```python
from build123d import *

# Parameters (mm, degrees)
ESQUISSE1_W        = 110
ESQUISSE1_H        = 50
ESQUISSE1_W_2      = 10
ESQUISSE1_H_2      = 10
BOSS_EXTRU_1_DEPTH = 4
CONG_1_R           = 3


with BuildPart() as part:
    # Esquisse1 → Boss.-Extru.1 (new body)
    with BuildSketch(Plane.XY):
        Rectangle(ESQUISSE1_W, ESQUISSE1_H)
        with Locations((-20, 0)):
            Rectangle(ESQUISSE1_W_2, ESQUISSE1_H_2, mode=Mode.SUBTRACT)
        with Locations((-40, 0)):
            Rectangle(ESQUISSE1_W_2, ESQUISSE1_H_2, mode=Mode.SUBTRACT)
        Rectangle(ESQUISSE1_W_2, ESQUISSE1_H_2, mode=Mode.SUBTRACT)
        with Locations((20, 0)):
            Rectangle(ESQUISSE1_W_2, ESQUISSE1_H_2, mode=Mode.SUBTRACT)
        with Locations((40, 0)):
            Rectangle(ESQUISSE1_W_2, ESQUISSE1_H_2, mode=Mode.SUBTRACT)
    extrude(amount=BOSS_EXTRU_1_DEPTH)

    # Congé1
    cong_1_edges = [part.edges().sort_by_distance(p)[0] for p in [
        (-55, 25, 2),
        (55, 25, 2),
        (55, -25, 2),
        (-55, -25, 2),
    ]]
    fillet(cong_1_edges, radius=CONG_1_R)


solid = part.part
```
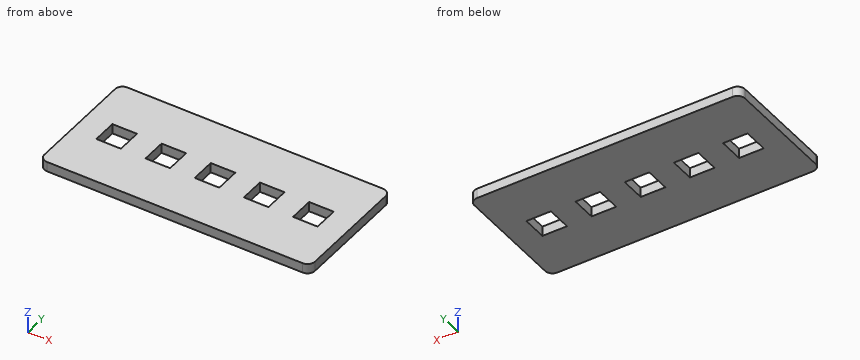
Source: CAD feature listing. Evaluate the final solid. Frame: model axes, mm. Round coordinates to 2 decimals unless told otherwise and drop trailing zeros. Loops run counter-clockwise (first coordinate to the right, second up) from the corner with the lowest first, then second, coordinate; pieces in that order, holes last.
(1) Section query A-A (x = -43). Output: boundary loops of the cut face in (y, z), and give its area (3 significant figures).
From the geometry:
outline: (-25, 0) - (-5, 0) - (-5, 4) - (-25, 4) - close; (5, 0) - (25, 0) - (25, 4) - (5, 4) - close
area: 160 mm2
(2) Material intervals for probe 1 along X at (y, z) = (4.5, 2.65); probe 2 along Y at (x, z) = (-23.5, 3.2), sorted ascending.
From the geometry:
probe 1: x = -55 to -45, -35 to -25, -15 to -5, 5 to 15, 25 to 35, 45 to 55
probe 2: y = -25 to -5, 5 to 25
(3) Section query B-B (y = -2.5). Output: boundary loops of the cut face in (x, z).
From the geometry:
outline: (-55, 0) - (-45, 0) - (-45, 4) - (-55, 4) - close; (-35, 0) - (-25, 0) - (-25, 4) - (-35, 4) - close; (-15, 0) - (-5, 0) - (-5, 4) - (-15, 4) - close; (5, 0) - (15, 0) - (15, 4) - (5, 4) - close; (25, 0) - (35, 0) - (35, 4) - (25, 4) - close; (45, 0) - (55, 0) - (55, 4) - (45, 4) - close
(4) Section query C-C (z = 2.25). Output: boundary loops of the cut face in (x, y).
From the geometry:
outline: (-55, -22) arc R3 ccw to (-52, -25) - (52, -25) arc R3 ccw to (55, -22) - (55, 22) arc R3 ccw to (52, 25) - (-52, 25) arc R3 ccw to (-55, 22) - close; hole (-45, -5) - (-35, -5) - (-35, 5) - (-45, 5) - close; hole (-25, -5) - (-15, -5) - (-15, 5) - (-25, 5) - close; hole (-5, -5) - (5, -5) - (5, 5) - (-5, 5) - close; hole (15, -5) - (25, -5) - (25, 5) - (15, 5) - close; hole (35, -5) - (45, -5) - (45, 5) - (35, 5) - close
